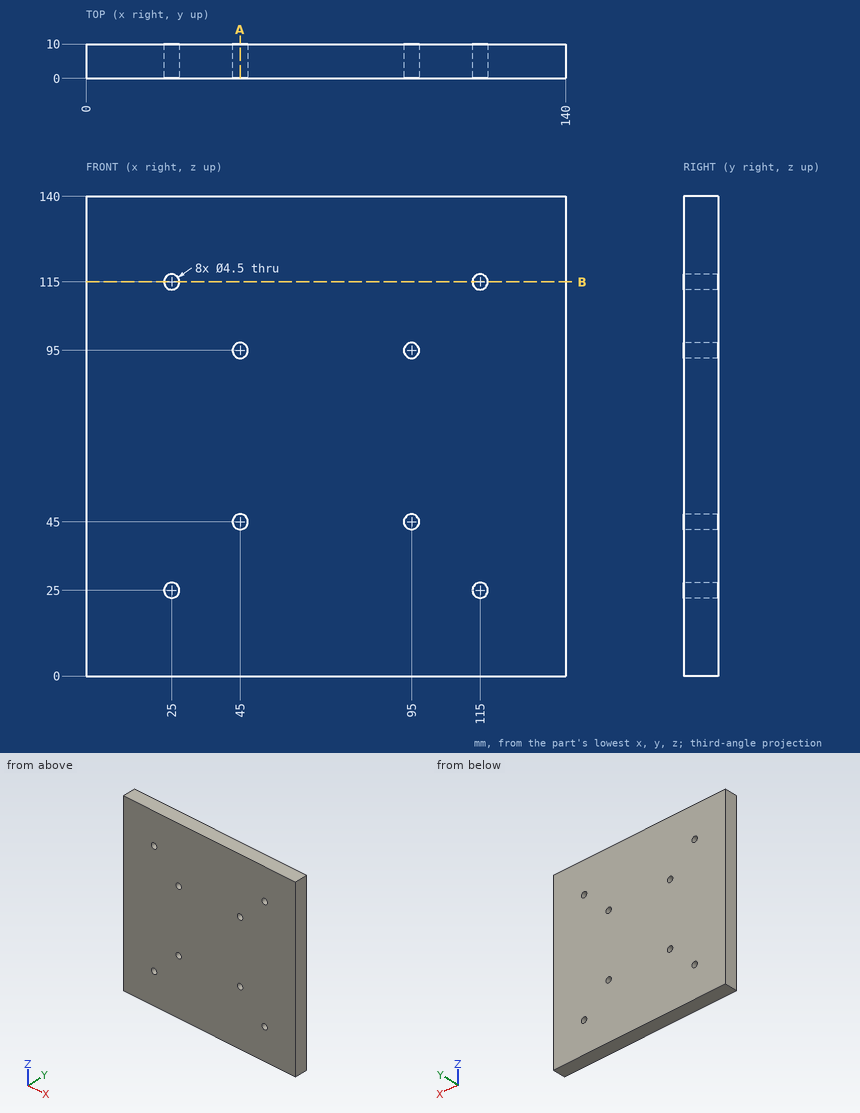
Geometry: see drawing. Coordinates: mm, zero at the bounding-box minimum. Round coordinates to 2 decimals unless told otherwise and drop trailing zeros. Write each loop counter-clockwise with the first axis right and the second up, starting at its lowest first coordinate (ties: lowest second). Pieces come first, ordered by that corner, then holes.
1) Contact query for flat-ended pins moving along their axis: P1, Ø7, axis at x = 115, z = 25, coming from the -Y side; P2, Ø4, axis at x = 95, z = 45, coming from the -Y side. Output: stop coordinate, or through.
2) Ray query, L1, parallel to Z at x = 115, y = 5; L2, parallel to Z at x = 45, y = 3. Return the intervals inside material, ascending.
3) Cut plane A-A (x = 45). Return the cut outline in (y, z), then the cut area to 3 significant figures.
4) Cut plane B-B (z = 115). Return the cut outline in (x, y).
Geometry says:
1. P1: stops at y = 0
1. P2: passes through
2. L1: z = 0 to 22.75, 27.25 to 112.75, 117.25 to 140
2. L2: z = 0 to 42.75, 47.25 to 92.75, 97.25 to 140
3. outline: (0, 0) - (10, 0) - (10, 42.75) - (0, 42.75) - close; (0, 47.25) - (10, 47.25) - (10, 92.75) - (0, 92.75) - close; (0, 97.25) - (10, 97.25) - (10, 140) - (0, 140) - close
3. area: 1,310 mm2
4. outline: (0, 0) - (22.75, 0) - (22.75, 10) - (0, 10) - close; (27.25, 0) - (112.75, 0) - (112.75, 10) - (27.25, 10) - close; (117.25, 0) - (140, 0) - (140, 10) - (117.25, 10) - close
